Build history of the part. All positions in model axes, mm. A direction names the side the tool comes from. Coordinates: 2 decimals unless noted, no trailing zeros. Loops run counter-clockwise (first coordinate to the right, second up) from the corner with the lowest first, then second, coordinate; pieces in that order, holes last. Notation, with made-up numbers: (56.25, 29.5) -> (98.25, 29.5) arc R9 cw to (98.25, 39.5) -> close; hole circle Ø3 at (29, 34). An arc over 180 degrees is marked (long way). One line per item, written item: value. Start each with the question number.
```python
from build123d import *

# Parameters (mm, degrees)
SKETCH1_W           = 24.5
SKETCH1_H           = 40.5
SKETCH1_W_2         = 20.5
SKETCH1_H_2         = 36.5
BOSS_EXTRUDE1_DEPTH = 27
SKETCH1_2_W         = 24.5
SKETCH1_2_H         = 40.5
SKETCH1_2_W_2       = 20.5
SKETCH1_2_H_2       = 36.5
BOSS_EXTRUDE2_DEPTH = 2
SKETCH2_W           = 9
SKETCH2_H           = 22
CUT_EXTRUDE1_DEPTH  = 2
CUT_EXTRUDE2_DEPTH  = 2
SKETCH4_W           = 27.5
SKETCH4_H           = 43.5
SKETCH4_W_2         = 24.5
SKETCH4_H_2         = 40.5
BOSS_EXTRUDE3_DEPTH = 29
SKETCH5_W           = 9
SKETCH5_H           = 1.5
CUT_EXTRUDE3_DEPTH  = 2


with BuildPart() as part:
    # Sketch1 → Boss-Extrude1 (new body)
    with BuildSketch(Plane.XY):
        Rectangle(SKETCH1_W, SKETCH1_H)
        Rectangle(SKETCH1_W_2, SKETCH1_H_2, mode=Mode.SUBTRACT)
    extrude(amount=BOSS_EXTRUDE1_DEPTH)

    # Sketch1<2> → Boss-Extrude2 (add)
    # profile 1 of 2: a face of its own
    with BuildSketch(Plane.XY):
        Rectangle(SKETCH1_2_W, SKETCH1_2_H)
        Rectangle(SKETCH1_2_W_2, SKETCH1_2_H_2, mode=Mode.SUBTRACT)
    # profile 2 of 2: a face of its own
    with BuildSketch(Plane.XY):
        Rectangle(SKETCH1_2_W_2, SKETCH1_2_H_2)
    extrude(amount=-BOSS_EXTRUDE2_DEPTH)

    # Sketch2 → Cut-Extrude1 (cut)
    with BuildSketch(Plane(origin=(0, 0, -2), x_dir=(-1, 0, 0), z_dir=(0, 0, -1))):
        with Locations((-5.75, -4.25)):
            Rectangle(SKETCH2_W, SKETCH2_H)
    extrude(amount=-CUT_EXTRUDE1_DEPTH, mode=Mode.SUBTRACT)

    # Sketch3 → Cut-Extrude2 (cut)
    with BuildSketch(Plane(origin=(0, 0, -2), x_dir=(-1, 0, 0), z_dir=(0, 0, -1))):
        Polygon((-11.75, 9.45), (-11.75, 8.25), (0.25, 8.25), (1.45, 8.25), (1.45, 9.45), align=None)
    extrude(amount=-CUT_EXTRUDE2_DEPTH, mode=Mode.SUBTRACT)

    # Sketch4 → Boss-Extrude3 (add)
    with BuildSketch(Plane(origin=(0, 0, -2), x_dir=(-1, 0, 0), z_dir=(0, 0, -1))):
        Rectangle(SKETCH4_W, SKETCH4_H)
        Rectangle(SKETCH4_W_2, SKETCH4_H_2, mode=Mode.SUBTRACT)
    extrude(amount=-BOSS_EXTRUDE3_DEPTH)

    # Sketch5 → Cut-Extrude3 (cut)
    with BuildSketch(Plane.XY):
        with Locations((5.75, 7.5)):
            Rectangle(SKETCH5_W, SKETCH5_H)
    extrude(amount=-CUT_EXTRUDE3_DEPTH, mode=Mode.SUBTRACT)


solid = part.part
```
Item 1: Drop a flat-ended pin along its axis: pin 1 Ø1 at (x, y) = (7, 15.5) entering from +Z. Give the stop position or say it passes through.
Item 2: Probe probe 1 along Y at (x, z) = (5, 3.5); probe 2 along X at (y, z) = (-12, 15.25); probe 3 along Z at (x, y) = (-2.75, -11.5). List the from-to ranges inside material, lowest first.
Item 3: Two-plate mould, pull along Y, no slides. Class faces 1 (the face through (10.25, 0, 13)), 2 (the face through (0, 0, -2)), 3 (the face through (0, -21.75, 12)): +Y half, -Y half, draft (parallel to the pull), parting line (faces both ways), or undercut.
Item 4: Band-saw the part on D-D, the plane x = -6.25. List the corners of the cut face in (y, z).
Item 5: Band-saw the part on B-B, the plane y = -6. List the corners of the cut face in (x, z).
Item 6: Tool access for faces 4 (the face through (11, 9, 0)), 5 (the face through (-2, 0, 0)), 6 (the face through (-1.45, 9, -1)), 7 (the face through (0, 21.75, 12)): list every direction of +Z, -Z, +X, -X, +Y, -Y with a clear straight run to the whole face (end or side of a thin tool).
Item 7: Band-saw the part on C-C, the plane z = 3.25. List the corners of the cut face in (x, y), and give its area (3 significant figures).
Item 8: Band-saw the part on A-A, the plane x = 0.5. List the corners of the cut face in (y, z), and give its area (3 significant figures).
Worked out:
1. pin 1: stops at z = 0
2. probe 1: y = -21.75 to -18.25, 18.25 to 21.75
2. probe 2: x = -13.75 to -10.25, 10.25 to 13.75
2. probe 3: z = -2 to 0
3. face 1: undercut
3. face 2: draft
3. face 3: -Y half
4. outline: (-21.75, -2) -> (21.75, -2) -> (21.75, 27) -> (18.25, 27) -> (18.25, 0) -> (-18.25, 0) -> (-18.25, 27) -> (-21.75, 27) -> close
5. outline: (-13.75, -2) -> (1.25, -2) -> (1.25, 0) -> (-10.25, 0) -> (-10.25, 27) -> (-13.75, 27) -> close; (10.25, -2) -> (13.75, -2) -> (13.75, 27) -> (10.25, 27) -> close
6. face 4: -Z
6. face 5: +Z
6. face 6: +Z, -Z
6. face 7: +Z, -Z, +X, -X, +Y
7. outline: (-13.75, -21.75) -> (13.75, -21.75) -> (13.75, 21.75) -> (-13.75, 21.75) -> close; hole (-10.25, -18.25) -> (10.25, -18.25) -> (10.25, 18.25) -> (-10.25, 18.25) -> close
7. area: 448 mm²
8. outline: (-21.75, -2) -> (8.25, -2) -> (8.25, 0) -> (-18.25, 0) -> (-18.25, 27) -> (-21.75, 27) -> close; (9.45, -2) -> (21.75, -2) -> (21.75, 27) -> (18.25, 27) -> (18.25, 0) -> (9.45, 0) -> close
8. area: 274 mm²
